Can you work these out from the model? Positions are in its coordinate system, mm. Give positions to 0.01 mm unless a question says otherwise; leave off trailing zeros. Loops run counter-clockwise (first coordinate to the right, second up) from the corner with the lowest first, then second, coordinate; pieces in that order, holes last. Notation, with made-up numbers: (-9.75, 6.25) - (25.25, 6.25) arc R19 cw to (25.25, 34.25) - close; hole circle Ø3 at (-26.75, 73.25). An arc over 180 degrees is marked (long way). Answer as a JSON object with one key per item and string values.
```python
from build123d import *

# Parameters (mm, degrees)
SKETCH1_R            = 43
SKETCH1_R_2          = 42.5
EXTRUDE_THIN1_DEPTH  = 35
EXTRUDE_THIN2_START  = -3.5
SKETCH2_R            = 44.1
SKETCH2_R_2          = 42.5
EXTRUDE_THIN2_DEPTH  = 3.5
FILLET1_R            = 1
FILLET1_OF_MIRROR1_R = 1


with BuildPart() as part:
    # Sketch1 → Extrude-Thin1 (new, symmetric)
    with BuildSketch(Plane.XY):
        Circle(SKETCH1_R)
        Circle(SKETCH1_R_2, mode=Mode.SUBTRACT)
    extrude(amount=EXTRUDE_THIN1_DEPTH, both=True)

    # Sketch2 → Extrude-Thin2 (add)
    with BuildSketch(Plane.XY.offset(35).offset(EXTRUDE_THIN2_START)):
        Circle(SKETCH2_R)
        Circle(SKETCH2_R_2, mode=Mode.SUBTRACT)
    extrude_thin2 = extrude(amount=EXTRUDE_THIN2_DEPTH)

    # Fillet1
    fillet1_edges = [part.edges().sort_by_distance(p)[0] for p in [
        (-44.1, 0, 35),
        (-44.1, 0, 31.5),
    ]]
    fillet(fillet1_edges, radius=FILLET1_R)

    # Mirror1: Extrude-Thin2 across plane
    add(extrude_thin2.mirror(Plane.XY))

    # Fillet1 of Mirror1
    fillet1_of_mirror1_edges = [part.edges().sort_by_distance(p)[0] for p in [
        (-44.1, 0, -35),
        (-44.1, 0, -31.5),
    ]]
    fillet(fillet1_of_mirror1_edges, radius=FILLET1_OF_MIRROR1_R)


solid = part.part
```
1) I'm going to push flat-ended pins straight in: P1, Ø4, axis at x = -6.5, z = -21, coming from the +Y side; P2, Ø2, axis at x = -34, z = -24, coming from the -Y side; P3, Ø6, axis at x = 16.5, z = 23, coming from the +Y side. Where does each tip first touch, or does it pass through?
Check sheet entries:
{"P1": "y = 42.76", "P2": "y = -27.57", "P3": "y = 40.83"}
2) Imagine slicing it at C-C on z = -22.5. Write out the boundary of the cut face in (x, y).
Check sheet entries:
{"outline": "circle Ø86 at (0, 0); hole circle Ø85 at (0, 0)"}
3) I need wall thicknesses on L1, parallel to Y at x = 0, z = 6; L2, parallel to Y at x = 29, z = 29.5; L3, parallel to X at y = -17, z = 18. Which ranges of each line are inside material? Lowest first, please.
Check sheet entries:
{"L1": "-43 to -42.5, 42.5 to 43", "L2": "-31.75 to -31.07, 31.07 to 31.75", "L3": "-39.5 to -38.95, 38.95 to 39.5"}
4) Imagine slicing it at A-A on y = 0. Write out the boundary of the cut face in (x, z), and give its area (3 significant figures).
Check sheet entries:
{"outline": "(-44.1, -34) arc R1 ccw to (-43.1, -35) - (-42.5, -35) - (-42.5, 35) - (-43.1, 35) arc R1 ccw to (-44.1, 34) - (-44.1, 32.5) arc R1 ccw to (-43.1, 31.5) - (-43, 31.5) - (-43, -31.5) - (-43.1, -31.5) arc R1 ccw to (-44.1, -32.5) - close; (42.5, -35) - (43.1, -35) arc R1 ccw to (44.1, -34) - (44.1, -32.5) arc R1 ccw to (43.1, -31.5) - (43, -31.5) - (43, 31.5) - (43.1, 31.5) arc R1 ccw to (44.1, 32.5) - (44.1, 34) arc R1 ccw to (43.1, 35) - (42.5, 35) - close", "area": "83.7 mm2"}
5) If we mould it in two halves opening along Z, with no side actions, what happens to faces 1 (the cylindrical face through (-5.598, 42.634, 0.441)), 2 (the cylindrical face through (-33.727, -25.861, -0.49)), 3 (the flat face through (31.72, -28.53, 35))? For each: released by +Z, released by -Z, zero draft, split by the parting line, or undercut.
Check sheet entries:
{"face 1": "undercut", "face 2": "zero draft", "face 3": "released by +Z"}
